Autodesk Inventor part; units mm, degrees
ref_plane "Work Plane1" through (2.2553, 0, 0) normal (0, 0, -1) x (1, 0, 0)
ref_plane "YZ Plane" through (0, 0, 0) normal (1, 0, 0) x (0, 1, 0)
ref_plane "XZ Plane" through (0, 0, 0) normal (0, 1, 0) x (-1, 0, 0)
sketch "Sketch1" plane through (0, 0, 0) normal (0, 0, 1) x (1, 0, 0)
  line L0 (-4, 0) -> (24, 0)
  line L1 (0, 0) -> (20, 0)
  line L2 (20, 0) -> (20, 1.75)
  line L3 (20, 1.75) -> (2.3, 1.75)
  line L4 (2.3, 1.75) -> (2.3, 1.75)
  line L5 (2.3, 1.75) -> (0.6, 3.45)
  line L6 (0.6, 3.45) -> (0, 3.45)
  line L7 (0, 3.45) -> (0, 0)
  line L8 (0, -0.69) -> (0, 4.14)
  dimension "d0" = 20
  dimension "d1" = 2.3
  dimension "d2" = 3.5
  dimension "d3" = 3.5
  dimension "d4" = 6.9
  dimension "d5" = 45
revolve "Body" add sketch "Sketch1" angle 360 about axis through (0, 0, 0) along (1, 0, 0)
sketch "Sketch2" plane through (0, 0, 0) normal (-1, 0, 0) x (0, 0, 1)
  circle A0 centre (0, 0) radius 3.45
  line L0 (-4.83, 0) -> (4.83, 0)
  line L1 (-3.45, 0) -> (-3.45, 0.6)
  line L2 (-3.45, 0.6) -> (3.45, 0.6)
  line L3 (3.45, 0) -> (3.45, 0.6)
  line L4 (-3.45, 0) -> (-3.45, -0.6)
  line L5 (-3.45, -0.6) -> (3.45, -0.6)
  line L6 (3.45, 0) -> (3.45, -0.6)
  dimension "d8" = 1.2
extrude "Slot" cut sketch "Sketch2" against normal blind 1.2 contours L0 A0 L2 | L6 L5 A0 | A0 L5 L0 | A0 L2 L3 | L1 L2 A0 | A0 L5 L4
thread "Thread"
chamfer "Chamfer1" distance 0.41 distance2 2.7 1 edges at (20, -1.75, 0) measured on face at (20, 0.4611, 1.0065)
ref_plane "Work Plane1" through (2.2553, 0, 0) normal (0, 0, -1) x (1, 0, 0)
equation "\"d8\" = SBR"
equation "\"d9\" = STI"
equation "\"d0\" = NLG"
equation "\"d1\" = KOH"
equation "\"d2\" = NND"
equation "\"d3\" = SED2"
equation "\"d4\" = KOD"
equation "\"d5\" = 0.5 * SEWI"
equation "\"d6\" = GEL"
equation "\"d14\" = -0.5 * GD2 + 0.5 * NND"
equation "\"d15\" = SPTZ"
equation "\"NND\" = 3.5"
equation "\"NLG\" = 20"
equation "\"GEL\" = 17.7"
equation "\"KOH\" = 2.3"
equation "\"KOD\" = 6.9"
equation "\"SBR\" = 1.2"
equation "\"STI\" = 1.2"
equation "\"GD2\" = 2.68"
equation "\"SED2\" = 3.5"
equation "\"SEWI\" = 90deg"
equation "\"SPTZ\" = 2.7"
equation "\"GUL\" = 0.61345 * PTC"
equation "\"THREADDIA\" = 3.5"
equation "\"TOA\" = 30deg"
equation "\"PTC\" = 0.6"
equation "\"GAL\" = 0.61345 * PTC"
equation "\"GD1\" = THREADDIA - 1.2269 * PTC"
properties part number "ANSI/ASME B18.6.5M - M3.5x0.6 x 20, SFCHTSTTM" material "Steel, Mild"
Design review of the part built by this model. Coordinates are the model's own, in mm. A direction names the side the tool comes from. Give positions to 0.01 mm unless a question says otherwise; leave off trailing zeros. Order: outer loops, then holes, each group sorted by start corner. A loop starts at its lowest first (then second) coordinate and runs counter-clockwise, first axis right, second up. Notation, with made-up numbers: (26, 23) - (34, 23) arc R31 ccw to (34, 61) - close; hole circle Ø2 at (74.25, 78.5). An arc over 180 degrees is marked (long way). Use a Markdown table: item, result. Add a question column.
(1) Add section C-C on x = 6.75. Give the boundary of the cut face in (y, z).
(2) Add section D-D on x = 17.75. Give the boundary of the cut face in (y, z).
(3) Add section B-B on z = 0. Give the boundary of the cut face in (x, y).
(4) Clearance check with flat-ended pins moving along their axes: P1, Ø2, axis at x = 12.5, z = 0.5, coming from the -Y side; P2, Ø4, axis at y = -1, z = -1.5, coming from the +X side; P3, Ø2, axis at x = 11, y = -0.5, coming from the +Z side; P4, Ø3, axis at x = 6, y = -1.5, coming from the -Z side. State where each tip first meets the part, or that it passes through.
(5) Mouldability with a two-part tool opening along Y and no side actions: class faces 4 (the face through (18.931, 1.433, -0.451)), 5 (the face through (20, 0, 0)), 6 (the face through (1.2, 0, 0)), 7 (the face through (1, -0.6, 0)) as +Y half, -Y half, draft (parallel to the pull), parting line (faces both ways), or undercut.
(6) Machinability: for faces 1 (the face through (9.695, 1.617, 0.67)), 2 (the face through (1, 0.6, 0)), 3 (the face through (0, -2, 0)), which of the approach directions +Z, -Z, +X, -X, +Y, -Y give a long, thin tool a straight path to every point of the face, cutting with its end or side? Answer none if there is none.
(7) Wall thickness on probe 1 along X at (y, z) = (-0.5, -0.5); probe 2 along Z at (x, y) = (12.75, 0); probe 3 along X at (y, z) = (-2, 0.75): over which ranges is each line inside the solid? List them lowest first. Write a range as [from, to].
(8) Add section A-A on y = 0. Give the boundary of the cut face in (x, z).
Report:
| question | item | result |
|---|---|---|
| 1 | outline | circle Ø3.5 at (0, 0) |
| 2 | outline | circle Ø3.36 at (0, 0) |
| 3 | outline | (0, -3.45) - (0.6, -3.45) - (2.3, -1.75) - (17.3, -1.75) - (20, -1.34) - (20, 1.34) - (17.3, 1.75) - (2.3, 1.75) - (0.6, 3.45) - (0, 3.45) - (0, 0.6) - (1.2, 0.6) - (1.2, -0.6) - (0, -0.6) - close |
| 4 | P1 | stops at y = -1.75 |
| 4 | P2 | stops at x = 20 |
| 4 | P3 | stops at z = 1.75 |
| 4 | P4 | stops at z = -1.75 |
| 5 | face 4 | parting line |
| 5 | face 5 | draft |
| 5 | face 6 | undercut |
| 5 | face 7 | undercut |
| 6 | face 1 | +X |
| 6 | face 2 | +Z, -Z, -X |
| 6 | face 3 | +Z, -Z, -X, +Y, -Y |
| 7 | probe 1 | x = [1.2, 20] |
| 7 | probe 2 | z = [-1.75, 1.75] |
| 7 | probe 3 | x = [0, 1.91] |
| 8 | outline | (1.2, -2.85) - (2.3, -1.75) - (17.3, -1.75) - (20, -1.34) - (20, 1.34) - (17.3, 1.75) - (2.3, 1.75) - (1.2, 2.85) - close |
